Verification items for the finished model (mm, model axes). Face numbers are marked on the shaded views. A direction names the side the tool comes from. Coordinates: 2 decimals unless noted, no trailing zeros. Loops run counter-clockwise (first coordinate to the right, second up) from the corner with the lowest first, then second, coordinate; pieces in that order, holes last.
Q1. Go/stop test with flat-tipped pins: P1, Ø1.2, axis at x = 24.5, y = 93.5, coming from the -Z side; P2, Ø3, axis at y = 66, z = 63, coming from the -X side; P3, Ø5, axis at y = 24.5, z = 23.5, coming from the +X side. Record where each tip stops, or that it passes through.
Q2. Access from +Z, -Z, +X, -X, +Y, -Y to the whole of each face (thin tool, end or side, straight path). Record for the marked faces 1, 2 and 3.
Q3. Material ranges on probe 1 along Y at (x, z) = (23.55, 73.5); probe 2 along X at (y, z) = (38, 69.5); probe 3 along Z at (x, y) = (23.55, 75.5), recorded low to high.
Q4. Sectioned sample at D-D (z = 35.5). Enter the section's corners in (x, y).
Q5. Sectioned sample at A-A (y = 9.5). Enter the section's corners in (x, z).
Q6. Mould release check, pull along Z, two halves, no side actions. Record for the marked faces 4, 5, 6 and 7: +Z half, -Z half, draft (parallel to the pull), parting line (faces both ways), or undercut.
Q7. Sectioned sample at B-B (y = 24.5). Count the separate pieces of the cut face and the enclosed holes in it, then the cut area to 3 significant figures.
Q8. Sectioned sample at C-C (x = 8.5). Enter the section's corners in (y, z), then the cut area to 3 significant figures.
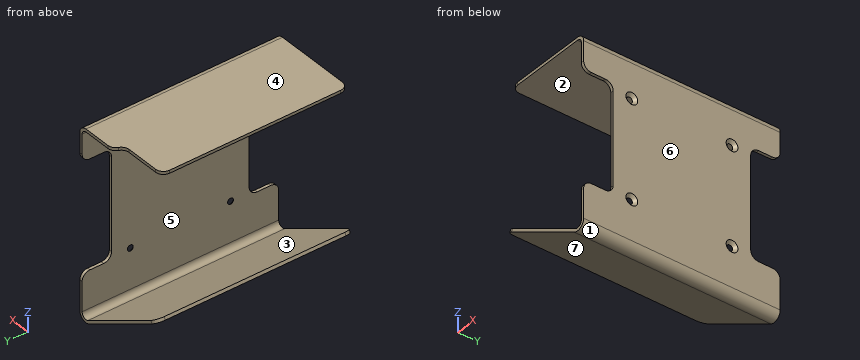
Autodesk Inventor part; units mm, degrees
ref_plane "YZ Plane" through (0, 0, 0) normal (1, 0, 0) x (0, 1, 0)
ref_plane "XZ Plane" through (0, 0, 0) normal (0, 1, 0) x (-1, 0, 0)
ref_plane "XY Plane" through (0, 0, 0) normal (0, 0, 1) x (1, 0, 0)
sketch "Sketch2" plane through (0, 0, 0) normal (0, 1, 0) x (-1, 0, 0)
  line L0 (-23.5, 25.6213) -> (-23.5, 95)
  line L1 (-23.5, 95) -> (-25, 95)
  line L2 (-25, 95) -> (-25, 25)
  line L3 (-25, 25) -> (0, 0)
  line L4 (0, 0) -> (25, 25)
  line L5 (23.5, 25.6213) -> (0, 2.1213)
  line L6 (0, 2.1213) -> (-23.5, 25.6213)
  line L7 (23.5, 25.6213) -> (25, 25)
  line L8 (25, 25) -> (-25, -3.8675)
  line L9 (-25, -3.8675) -> (-25, 25)
  line L10 (-23.5, 25.6213) -> (-23.5, -1.2694)
  line L11 (-23.5, -1.2694) -> (24.25, 26.299)
  line L12 (24.25, 26.299) -> (25, 25)
  point P0 (24.5092, 24.5092)
  dimension "d11" = 1.5
  dimension "d18" = 1.5
  dimension "d19" = 1.5
  dimension "d27" = 70
  dimension "d28" = 50
  dimension "d29" = 135
  dimension "d47" = 60
  dimension "d48" = 1.5
extrude "Extrusion2" add sketch "Sketch2" along normal blind 100 contours L10 L3 L2 L1 L0 | L11 L12 L7 L5 L8 L6 | L6 L8 L3 L11 | L10 L11 L3 L8 L9 | L5 L7 L8
fillet "Fillet3" radius 2.5 1 edges at (23.5, 50, -1.2694)
sketch "Sketch7" plane through (23.5, 0, 95) normal (-1, 0, 0) x (0, 0, 1)
  line L0 (0, 0) -> (0, 100)
  line L1 (0, 0) -> (-1.5, 0)
  line L2 (-1.5, 0) -> (-1.5, 100)
  line L3 (-1.5, 100) -> (0, 100)
  line L4 (0, 100) -> (0, 0)
  line L5 (-91.9393, 100) -> (0, 100)
  point P0 (-95, 0)
  dimension "d49" = 1.5
extrude "Extrusion7" add sketch "Sketch7" along normal blind 45
fillet "Fillet12" radius 4 2 edges at (25, 50, 95) (25, 50, -3.8675)
fillet "Fillet13" radius 2.5 1 edges at (23.5, 50, 93.5)
sketch "Sketch8" plane through (23.5, 0, 3.0607) normal (-1, 0, 0) x (0, 0, 1)
  line L0 (18.9393, 0) -> (73.9393, 0)
  line L1 (73.9393, 0) -> (73.9393, 15)
  line L2 (73.9393, 15) -> (18.9393, 15)
  line L3 (18.9393, 15) -> (18.9393, 0)
  line L4 (18.9393, 85) -> (73.9393, 85)
  line L5 (73.9393, 85) -> (73.9393, 100)
  line L6 (73.9393, 100) -> (18.9393, 100)
  line L7 (18.9393, 100) -> (18.9393, 85)
  line L8 (0, 100) -> (87.9393, 100)
  line L9 (0, 0) -> (87.9393, 0)
  line L10 (91.9393, 0) -> (91.9393, 100)
  point P0 (-3.0607, 0)
  dimension "d54" = 15
  dimension "d55" = 55
  dimension "d58" = 18
extrude "Extrusion8" cut sketch "Sketch8" against normal through all
sketch "Sketch9" plane through (-21.5, 0, 95) normal (0, 0, 1) x (1, 0, 0)
  line L0 (0, 100) -> (0, 0)
  line L1 (0, 100) -> (25, 100)
  line L2 (25, 100) -> (25, 95)
  line L3 (25, 95) -> (0, 95)
  line L4 (0, 95) -> (0, 100)
  point P0 (21.5, 0)
  dimension "d60" = 5
  dimension "d61" = 25
extrude "Extrusion9" cut sketch "Sketch9" against normal blind 35
fillet "Fillet14" radius 4 14 edges at (24.25, 85, 77) (24.25, 85, 22) (24.25, 100, 22) (24.25, 100, 77) (24.25, 15, 22) (24.25, 0, 22) (24.25, 15, 77) (24.25, 0, 77) (-21.5, 95, 94.25) (3.5, 95, 94.25) (3.5, 100, 94.25) (-21.5, 0, 94.25) (-24.625, 0, 25.6495) (-24.625, 100, 25.6495)
sketch "Sketch10" plane through (25, 0, 3.0607) normal (1, 0, 0) x (0, 0, -1)
  circle A0 centre (-70.4393, 75.5) radius 1.5
  circle A1 centre (-20.4393, 75.5) radius 1.5
  circle A2 centre (-70.4393, 24.5) radius 1.5
  circle A3 centre (-20.4393, 24.5) radius 1.5
  line L0 (-91.9393, 100) -> (-91.9393, 0)
  line L1 (-91.9393, 4) -> (-91.9393, 91)
  line L2 (-87.9393, 100) -> (-77.9393, 100)
  point P0 (3.0607, 0)
  dimension "d64" = 3
  dimension "d65" = 50
  dimension "d66" = 51
  dimension "d70" = 24.5
  dimension "d71" = 21.5
extrude "Extrusion10" cut sketch "Sketch10" against normal blind 5
chamfer "Chamfer1" distance 1.5 angle 45 4 edges at (25, 75.5, 75) (25, 75.5, 25) (25, 24.5, 25) (25, 24.5, 75)
properties part number "armor"
Geometry check:
1. P1: stops at z = 0.31
1. P2: stops at x = 23.5
1. P3: stops at x = 24.5
2. face 1: -Z, +Y, -Y
2. face 2: -X, +Y, -Y
2. face 3: +Y, -Y
3. probe 1: y = 14.97 to 22.95, 26.05 to 73.95, 77.05 to 85.03
3. probe 2: x = 23.5 to 25
3. probe 3: z = -0.02 to 21.95, 25.05 to 71.95, 75.05 to 94.08
4. outline: (23.5, 15) - (25, 15) - (25, 85) - (23.5, 85) - close
5. outline: (-25, 25) - (19, -0.4) arc R4 ccw to (25, 3.06) - (25, 22) - (23.5, 22) - (23.5, 3.06) arc R2.5 cw to (19.75, 0.9) - (-24.25, 26.3) - close; (-21.5, 93.5) - (21, 93.5) arc R2.5 cw to (23.5, 91) - (23.5, 77) - (25, 77) - (25, 91) arc R4 ccw to (21, 95) - (-21.5, 95) - close
6. face 4: +Z half
6. face 5: undercut
6. face 6: draft
6. face 7: -Z half
7. separate pieces: 3
7. enclosed holes: 0
7. area: 276 mm2
8. outline: (0, 5.66) - (100, 5.66) - (100, 7.39) - (0, 7.39) - close; (0, 93.5) - (100, 93.5) - (100, 95) - (0, 95) - close
8. area: 323 mm2
